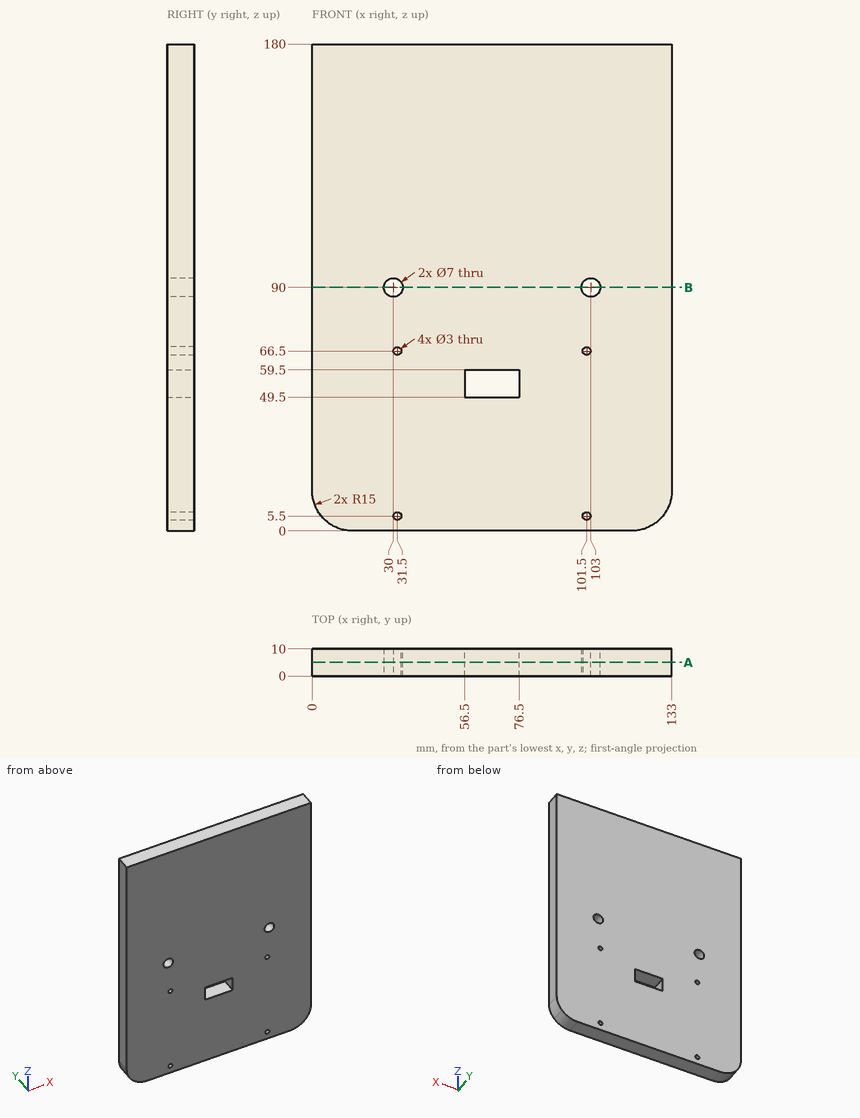
Part print with two shaded views. Sizes in mm from the minimum x, y, z corner. Give positions to 0.01 mm unless a question says otherwise; leave off trailing zeros. Order: outer loops, then holes, each group sorted by start corner. A loop starts at its lowest first (then second) coordinate and runs counter-clockwise, first axis right, second up.
(1) Drill centre lines: L1, parallel to X at y = 4.25, z = 90; L2, parallel to X at y = 4.5, z = 66.5; L3, parallel to Z at x = 101.5, y = 7.75. Where is each one in solid material? Low to high.
(2) Flat gauge pin, fed straight in: pin 1 (1.8 mm diameter, centred on x = 101.5, z = 5.5, fed in from -Y). Where does the tip first touch, or does it go through?
(3) Saw through at A-A, the plane y = 5. Give the cut face in (x, z).
(4) Saw through at B-B, the plane z = 90. Give the cut face in (x, y).
Results found:
1. L1: x = 0 to 26.5, 33.5 to 99.5, 106.5 to 133
1. L2: x = 0 to 30, 33 to 100, 103 to 133
1. L3: z = 0 to 4, 7 to 65, 68 to 86.84, 93.16 to 180
2. pin 1: passes through
3. outline: (0, 15) arc R15 ccw to (15, 0) - (118, 0) arc R15 ccw to (133, 15) - (133, 180) - (0, 180) - close; hole circle Ø7 at (30, 90); hole circle Ø3 at (31.5, 5.5); hole circle Ø3 at (31.5, 66.5); hole (56.5, 49.5) - (76.5, 49.5) - (76.5, 59.5) - (56.5, 59.5) - close; hole circle Ø7 at (103, 90); hole circle Ø3 at (101.5, 5.5); hole circle Ø3 at (101.5, 66.5)
4. outline: (0, 0) - (26.5, 0) - (26.5, 10) - (0, 10) - close; (33.5, 0) - (99.5, 0) - (99.5, 10) - (33.5, 10) - close; (106.5, 0) - (133, 0) - (133, 10) - (106.5, 10) - close
